Here's how the part is built. I have some questions about the finished solid (model axes, mm). Face numbers are marked on the shaded views. Round coordinates to 2 decimals unless told otherwise and drop trailing zeros. Order: outer loops, then holes, each group sorted by start corner. A loop starts at its lowest first (then second) coordinate and runs counter-clockwise, first axis right, second up. Notation, with made-up numbers: (20, 89.25) -> (62, 89.25) arc R18 cw to (62, 122.25) -> close; hole circle Ø7 at (59.25, 75.25). An arc over 180 degrees is marked (long way). Answer in a Markdown table with one row per item.
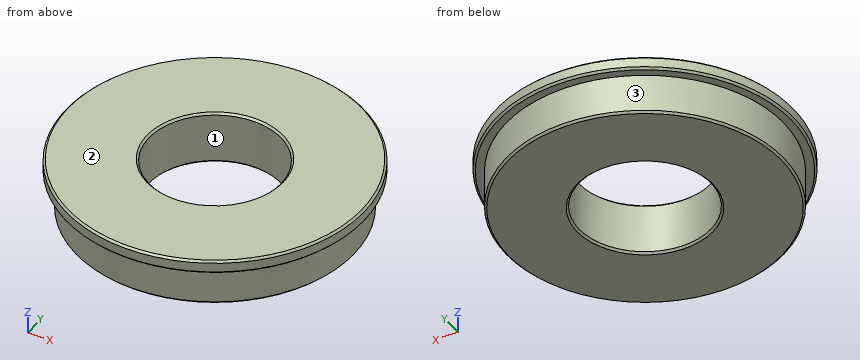
```python
from build123d import *

# Parameters (mm, degrees)
SKETCH_1_R      = 21
SKETCH_1_R_2    = 10
EXTRUDE_1_DEPTH = 4
EXTRUDE_START   = -2
SKETCH_2_R      = 22.5
SKETCH_2_R_2    = 10
EXTRUDE_2_DEPTH = 2
CHAMFER_1_SIZE  = 0.3


with BuildPart() as part:
    # 草图1 → 凸台-拉伸1 (new, symmetric)
    with BuildSketch(Plane.XY):
        Circle(SKETCH_1_R)
        Circle(SKETCH_1_R_2, mode=Mode.SUBTRACT)
    extrude(amount=EXTRUDE_1_DEPTH, both=True)

    # 草图2 → 凸台-拉伸2 (add)
    with BuildSketch(Plane.XY.offset(4).offset(EXTRUDE_START)):
        Circle(SKETCH_2_R)
        Circle(SKETCH_2_R_2, mode=Mode.SUBTRACT)
    extrude(amount=EXTRUDE_2_DEPTH)

    # 倒角1
    chamfer_1_edges = [part.edges().sort_by_distance(p)[0] for p in [
        (-22.5, 0, 4),
        (-22.5, 0, 2),
        (-21, 0, -4),
        (-10, 0, -4),
        (-10, 0, 4),
    ]]
    chamfer(chamfer_1_edges, length=CHAMFER_1_SIZE)


solid = part.part
```
1. We'd pull the mould along Y, two halves only. Please class the marked faces 1, 2 and 3: released by +Y, released by -Y, zero draft, split by the parting line, or undercut.
Numbers:
| item | result |
|---|---|
| face 1 | undercut |
| face 2 | zero draft |
| face 3 | split by the parting line |
2. Suppose I cut it at C-C on z = -3. Write out the boundary of the cut face in (x, y), then the cut area to 3 significant figures.
Numbers:
| item | result |
|---|---|
| outline | circle Ø42 at (0, 0); hole circle Ø20 at (0, 0) |
| area | 1,070 mm2 |
3. For pin 1 Ø4 at (x, z) = (12, -1) entering from -Y; pin 2 Ø3 at (x, z) = (-11.5, 1.5) entering from -Y; pin 3 Ø1.5 at (x, z) = (8.5, -0.5) entering from -Y, each with a flat end and sliding along its axis, tell me the tip position at first contact or that it passes through.
Numbers:
| item | result |
|---|---|
| pin 1 | stops at y = -18.47 |
| pin 2 | stops at y = -20.04 |
| pin 3 | stops at y = -19.52 |
4. Suppose I cut it at A-A on y = 0. Write out the boundary of the cut face in (x, z).
Numbers:
| item | result |
|---|---|
| outline | (-22.5, 2.3) -> (-22.2, 2) -> (-21, 2) -> (-21, -3.7) -> (-20.7, -4) -> (-10.3, -4) -> (-10, -3.7) -> (-10, 3.7) -> (-10.3, 4) -> (-22.2, 4) -> (-22.5, 3.7) -> close; (10, -3.7) -> (10.3, -4) -> (20.7, -4) -> (21, -3.7) -> (21, 2) -> (22.2, 2) -> (22.5, 2.3) -> (22.5, 3.7) -> (22.2, 4) -> (10.3, 4) -> (10, 3.7) -> close |
5. Please list where these lines run through material, in increasing order: line 1 along Y through (x, z) = (0, -0.25); line 2 along Z through (x, y) = (-7, -20); line 3 along Y through (x, z) = (-5, 2.5).
Numbers:
| item | result |
|---|---|
| line 1 | y = -21 to -10, 10 to 21 |
| line 2 | z = 2 to 4 |
| line 3 | y = -21.94 to -8.66, 8.66 to 21.94 |
